Could you check a few things on this drawing? It's one solid part, dimensions in mm from its lowest x, y, z. A direction names the side the tool comes from. Give positions to 0.01 mm unless a question says otherwise; leave off trailing zeros. Loops run counter-clockwise (first coordinate to the right, second up) from the corner with the lowest first, then second, coordinate; pieces in that order, holes last. Notation, with made-up numbers: (-15, 86.5) - (-2, 86.5) arc R19 cw to (-2, 106.5) - close; hole circle Ø10 at (-12, -37.75). An arc over 180 degrees is marked (long way). Use CSV: the item, a comma, the result in double quotes.
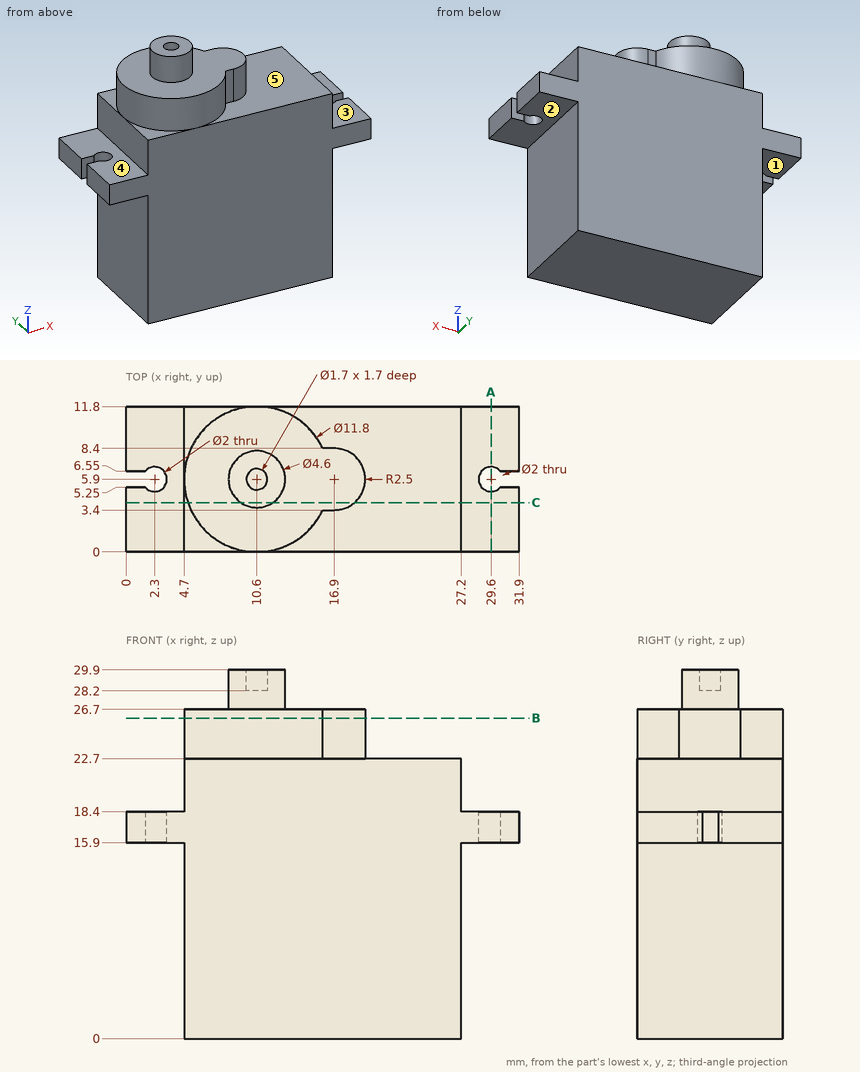
1) Suppose I cut it at B-B (z = 26). Please give me the cut outline in (x, y), plus the area to 3 significant figures.
Answer below:
outline,"(15.94, 3.4) - (16.9, 3.4) arc R2.5 ccw to (16.9, 8.4) - (15.94, 8.4) arc R5.9 ccw (long way) to start"
area,"122 mm2"
2) Which directions (+Z, -Z, +X, -X, +Y, -Y) give clear straight access to the entire face, cutting with the end or side of a thin tool? Please do the marked faces 1, 2, 3, 4 and 5.
Answer below:
face 1,"-Z, -X, +Y, -Y"
face 2,"-Z, +X, +Y, -Y"
face 3,"+Z, +X, +Y, -Y"
face 4,"+Z, -X, +Y, -Y"
face 5,"+Z, +X"
3) I need wall thicknesses on line 1 along Y through (x, z) = (2.3, 16.95); line 2 along X through (y, z) = (8.5, 2); line 3 along Z through (x, y) = (19, 7.5). Which ranges of each line are inside material? Lowest first, please.
Answer below:
line 1,"y = 0 to 4.9, 6.9 to 11.8"
line 2,"x = 4.7 to 27.2"
line 3,"z = 0 to 22.7"
4) Suppose I cut it at A-A (x = 29.6). Please give me the cut outline in (y, z).
Answer below:
outline,"(0, 15.9) - (4.9, 15.9) - (4.9, 18.4) - (0, 18.4) - close; (6.9, 15.9) - (11.8, 15.9) - (11.8, 18.4) - (6.9, 18.4) - close"
5) I'm going to push flat-ended pins straight in: P1, Ø1.5, axis at y = 8, z = 6, coming from the -X side; P2, Ø1, axis at x = 22, y = 8, coming from the -Z side; P3, Ø3.5, axis at y = 6.5, z = 10.5, coming from the +X side; P4, Ø3, axis at x = 8, y = 2, coming from the +Z side. Where does each tip first touch, or does it pass through?
Answer below:
P1,"stops at x = 4.7"
P2,"stops at z = 0"
P3,"stops at x = 27.2"
P4,"stops at z = 26.7"
6) Suppose I cut it at C-C (y = 4). Please give me the cut outline in (x, z), plus the area to 3 significant figures.
Answer below:
outline,"(0, 15.9) - (4.7, 15.9) - (4.7, 0) - (27.2, 0) - (27.2, 15.9) - (31.9, 15.9) - (31.9, 18.4) - (27.2, 18.4) - (27.2, 22.7) - (18.52, 22.7) - (18.52, 26.7) - (11.9, 26.7) - (11.9, 29.9) - (9.3, 29.9) - (9.3, 26.7) - (5.01, 26.7) - (5.01, 22.7) - (4.7, 22.7) - (4.7, 18.4) - (0, 18.4) - close"
area,"597 mm2"
